The listing builds one solid part. Answer for the finished solid, in the listing's coordinates (mm). A direction names the side the tool comes from. Round coordinates to 2 decimals unless told otherwise and drop trailing zeros. Loops run counter-clockwise (first coordinate to the right, second up) from the corner with the lowest first, then second, coordinate; pieces in that order, holes last. Notation, with made-up numbers: (81.5, -24.5) - (95.5, -24.5) arc R25 ccw to (95.5, -0.5) - close; hole circle Ø4 at (-24, -30). An arc over 180 degrees is marked (long way). One line per item, written item: value.
```python
from build123d import *

# Parameters (mm, degrees)
F0_W     = 300
F0_H     = 20
F1_DEPTH = 3
F2_R     = 2.5
F3_DEPTH = 3
F4_W     = 300
F4_H     = 3
F5_DEPTH = 15
F6_R     = 3


with BuildPart() as f1:
    # F0 (on Top) → F1 (new body)
    with BuildSketch(Plane.XY):
        Rectangle(F0_W, F0_H)
    extrude(amount=F1_DEPTH)

    # F2 (on face) → F3 (cut)
    with BuildSketch(Plane.XY.offset(3)):
        with Locations((-120, 2)):
            Circle(F2_R)
        with Locations((-120, -5)):
            Circle(F2_R)
        with Locations((-140, 0)):
            Circle(F2_R)
        Circle(F2_R)
        with Locations((140, 0)):
            Circle(F2_R)
    extrude(amount=-F3_DEPTH, mode=Mode.SUBTRACT)

    # F4 (on face) → F5 (join)
    with BuildSketch(Plane.XY.offset(3)):
        with Locations((0, 8.5)):
            Rectangle(F4_W, F4_H)
    extrude(amount=F5_DEPTH)

    # F6
    f6_edges = [f1.edges().sort_by_distance(p)[0] for p in [
        (0, 10, 0),
    ]]
    fillet(f6_edges, radius=F6_R)


solid = f1.part
```
1) Each of these flat-tipped pins is pushed along its axis until it touches: pin 1 Ø8 at (x, y) = (-140, 0) entering from +Z; pin 2 Ø2 at (x, z) = (-63.5, 13) entering from -Y. Where does it stop, or does it pass through?
Final values:
pin 1: z = 3
pin 2: y = 7
2) A cutting plane is placed at A-A on x = 140. Give the vertices of the cut face in (y, z), and give its area (3 significant figures).
Final values:
outline: (-10, 0) - (-2.5, 0) - (-2.5, 3) - (-10, 3) - close; (2.5, 0) - (7, 0) arc R3 ccw to (10, 3) - (10, 18) - (7, 18) - (7, 3) - (2.5, 3) - close
area: 88.1 mm2
3) A cutting plane is placed at B-B on y = -5. Give the vertices of the cut face in (x, z).
Final values:
outline: (-150, 0) - (-122.5, 0) - (-122.5, 3) - (-150, 3) - close; (-117.5, 0) - (150, 0) - (150, 3) - (-117.5, 3) - close
4) For faces 1 (the cylindrical face through (142.385, 0.751, 1.521)), 2 (the flat face through (-2, -3, 3)), determine the directions among +Z, -Z, +X, -X, +Y, -Y from which every point of the face is accessible in a straight line to the end or side of a thin tool.
Final values:
face 1: +Z, -Z
face 2: +Z, +X, -X, -Y
5) A cutting plane is placed at D-D on x = 95.5. Give the vertices of the cut face in (y, z), and give its area (3 significant figures).
Final values:
outline: (-10, 0) - (7, 0) arc R3 ccw to (10, 3) - (10, 18) - (7, 18) - (7, 3) - (-10, 3) - close
area: 103 mm2
6) A cutting plane is placed at C-C on x = -120. Give the vertices of the cut face in (y, z).
Final values:
outline: (-10, 0) - (-7.5, 0) - (-7.5, 3) - (-10, 3) - close; (-2.5, 0) - (-0.5, 0) - (-0.5, 3) - (-2.5, 3) - close; (4.5, 0) - (7, 0) arc R3 ccw to (10, 3) - (10, 18) - (7, 18) - (7, 3) - (4.5, 3) - close
7) For a pull along Y with two mould halves and no side action, classify faces 3 (the flat face through (-2, 7, 10)), 4 (the flat face through (-2, 10, 10)), 5 (the flat face through (150, 3, 2)), 6 (the cylindrical face through (-117.615, -4.249, 1.521)) as released by +Y, released by -Y, zero draft, split by the parting line, or undercut.
Final values:
face 3: released by -Y
face 4: released by +Y
face 5: zero draft
face 6: undercut
8) Consider L1, parallel to Y at x = -120, z = 1.2; L2, parallel to Y at x = -122, z = 6; L3, parallel to Z at x = -11.5, y = -5.5. Determine where each line is inside the solid, lowest interval first.
Final values:
L1: -10 to -7.5, -2.5 to -0.5, 4.5 to 9.4
L2: 7 to 10
L3: 0 to 3
